Model file for the job. Use its own axes, mm. A direction names the side the tool comes from. Give positions to 0.01 mm unless a question says otherwise; leave off trailing zeros. Loops run counter-clockwise (first coordinate to the right, second up) from the corner with the lowest first, then second, coordinate; pieces in that order, holes last. Notation, with made-up numbers: M 39.5,-3.5 L 96.5,-3.5 A23 cw 96.5,25.5 Z; hole C 84.25,79.5 d3. An arc over 180 degrees is marked long. Answer in a Markdown table with one row per item.
```python
from build123d import *

# Parameters (mm, degrees)
SKETCH_1_W                  = 3
SKETCH_1_H                  = 11
HOLE_WIZARD_M22_D           = 2
HOLE_WIZARD_M22_CSINK_D     = 4.4
HOLE_WIZARD_M22_CSINK_ANGLE = 90
PATTERN_CIRCULAR_2_COUNT    = 4
SKETCH_6_R                  = 3.5
EXTRUDE_1_DEPTH             = 17
SKETCH_7_R                  = 14
EXTRUDE_2_DEPTH             = 3
CUT_EXTRUDE_1_REACH         = 32.348
SKETCH_8_R                  = 1
PATTERN_CIRCULAR_3_COUNT    = 4


with BuildPart() as part:
    # Sketch 1 → Revolve 1 (revolve)
    with BuildSketch(Plane.XY, mode=Mode.PRIVATE) as revolve_1_sk:
        with Locations((5.5, 5.5)):
            Rectangle(SKETCH_1_W, SKETCH_1_H)
    revolve(revolve_1_sk.sketch.rotate(Axis((0, 0, 0), (1, 0, 0)), 90), axis=Axis((0, 0, 0), (1, 0, 0)))

    # Hole Wizard M22 (through all)
    with Locations(Plane(origin=(7, 0, 0), x_dir=(0, 0, -1), z_dir=(1, 0, 0))):
        with Locations((-2.933383142, 5.234048466)):
            hole_wizard_m22 = CounterSinkHole(HOLE_WIZARD_M22_D / 2, HOLE_WIZARD_M22_CSINK_D / 2, counter_sink_angle=HOLE_WIZARD_M22_CSINK_ANGLE)

    # Pattern Circular 2: Hole Wizard M22 ×4 about axis
    pattern_circular_2_axis = Axis((0, 0, 0), (1, 0, 0))
    for i in range(1, PATTERN_CIRCULAR_2_COUNT):
        add(hole_wizard_m22.rotate(pattern_circular_2_axis, i * 360 / PATTERN_CIRCULAR_2_COUNT), mode=Mode.SUBTRACT)

    # Sketch 6 → Extrude 1 (add)
    with BuildSketch(Plane(origin=(7, 0, 0), x_dir=(0, 0, -1), z_dir=(1, 0, 0))):
        with Locations(Location((0, 0, 0), (0, 0, 180))):
            Circle(SKETCH_6_R)
    extrude(amount=EXTRUDE_1_DEPTH)

    # Sketch 7 → Extrude 2 (add)
    with BuildSketch(Plane(origin=(24, 0, 0), x_dir=(0, 0, -1), z_dir=(1, 0, 0))):
        Circle(SKETCH_7_R)
    extrude(amount=EXTRUDE_2_DEPTH)

    # Sketch 8 → Cut-Extrude 1 (cut, up to next)
    with BuildSketch(Plane(origin=(27, 0, 0), x_dir=(0, 0, -1), z_dir=(1, 0, 0)), mode=Mode.PRIVATE) as cut_extrude_1_sk1:
        with Locations((-5.499090834, 7.5)):
            Circle(SKETCH_8_R)
    cut_extrude_1_tool1 = extrude(cut_extrude_1_sk1.sketch, amount=-CUT_EXTRUDE_1_REACH, mode=Mode.PRIVATE) & part.part
    cut_extrude_1 = cut_extrude_1_tool1.solids().sort_by_distance((27, 7.5, 5.499091))[0]
    add(cut_extrude_1, mode=Mode.SUBTRACT)

    # Pattern Circular 3: Cut-Extrude 1 ×4 about axis
    pattern_circular_3_axis = Axis((0, 0, 0), (1, 0, 0))
    for i in range(1, PATTERN_CIRCULAR_3_COUNT):
        add(cut_extrude_1.rotate(pattern_circular_3_axis, i * 360 / PATTERN_CIRCULAR_3_COUNT), mode=Mode.SUBTRACT)


solid = part.part
```
Q1. Saw through at C-C (y = 0). Give the cut face in (x, z).
Reported:
| item | result |
|---|---|
| outline | M 4,-11 L 7,-11 L 7,-3.5 L 24,-3.5 L 24,-14 L 27,-14 L 27,14 L 24,14 L 24,3.5 L 7,3.5 L 7,11 L 4,11 Z |
Q2. Probe probe 1 along X at (y, z) = (0.75, -8.25); probe 2 along X at (y, z) = (6, 3.5); probe 3 along Z at (x, y) = (5.25, -4.75). List the from-to ranges inside material, lowest first.
Reported:
| item | result |
|---|---|
| probe 1 | 4 to 7, 24 to 27 |
| probe 2 | 24 to 27 |
| probe 3 | -9.92 to -3.81, -2.06 to 9.92 |
Q3. 3-axis set-ups, long thin cutter, end or side, ignore diameter. For faces 1 (the face through (4.887, 4.347, 3.395)), 2 (the face through (25.479, -5.362, -12.932)), 3 (the face through (7, -2.6, 2.6)), 4 (the face through (25.521, 4.545, -7.8)), 5 (the face through (27, 0, 0)): which of +Z, -Z, +X, -X, +Y, -Y reach the whole face in a straight line?
Reported:
| item | result |
|---|---|
| face 1 | -X |
| face 2 | +X, -X |
| face 3 | none |
| face 4 | +X |
| face 5 | +Z, -Z, +X, +Y, -Y |
Q4. Mould opens along Z. For faces 6 (the face through (4.887, 3.395, -4.347)), 7 (the face through (5.52, 10.74, -2.38)), 8 (the face through (4, 0, 0)) say: released by +Z, released by -Z, zero draft, split by the parting line, or undercut.
Reported:
| item | result |
|---|---|
| face 6 | undercut |
| face 7 | split by the parting line |
| face 8 | zero draft |
Q5. Drop flat-ended pins along their axis: pin 1 (1.2 mm diameter, centred on y = -7.5, z = -5.5, fed in from +X); pin 2 (12 mm diameter, centred on x = 15, y = 10.5, fed in from +Z); pin 3 (1.6 mm diameter, centred on y = -5.23, z = -2.93, fed in from -X); pin 4 (3 mm diameter, centred on x = 23, z = 9.5, fed in from -Y). Give the stop position or say it passes through.
Reported:
| item | result |
|---|---|
| pin 1 | x = 7 |
| pin 2 | through |
| pin 3 | x = 24 |
| pin 4 | y = -11.21 |
Q6. Saw through at D-D (z = 0.25). Give the cut face in (x, y), and give its area (3 significant figures).
Reported:
| item | result |
|---|---|
| outline | M 4,-11 L 7,-11 L 7,-3.49 L 24,-3.49 L 24,-14 L 27,-14 L 27,14 L 24,14 L 24,3.49 L 7,3.49 L 7,11 L 4,11 Z |
| area | 269 mm² |
Q7. Saw through at B-B (x = 25). Give the cut face in (y, z).
Reported:
| item | result |
|---|---|
| outline | C 0,0 d28; hole C -7.5,-5.5 d2; hole C -5.5,7.5 d2; hole C 5.5,-7.5 d2; hole C 7.5,5.5 d2 |
Q8. Saw through at A-A (y = 9). Give the cut face in (x, z).
Reported:
| item | result |
|---|---|
| outline | M 4,-6.32 L 7,-6.32 L 7,6.32 L 4,6.32 Z; M 24,-10.72 L 27,-10.72 L 27,10.72 L 24,10.72 Z |
